Geometry check sheet. Reference: the model listing, model coordinates, mm. Face numbers are marked on the shaded views. A direction names the side the tool comes from. Give positions to 0.01 mm unless a question says otherwise; leave off trailing zeros. Order: outer loops, then holes, each group sorted by start corner. A loop starts at its lowest first (then second) coordinate and runs counter-clockwise, first axis right, second up. Notation, with made-up numbers: M 34.5,36 L 66.5,36 A32 cw 66.5,73 Z; hole C 9.25,59.5 d1. An arc over 180 degrees is marked long. One line per question, with ' | ' between items. Start each with the question number.
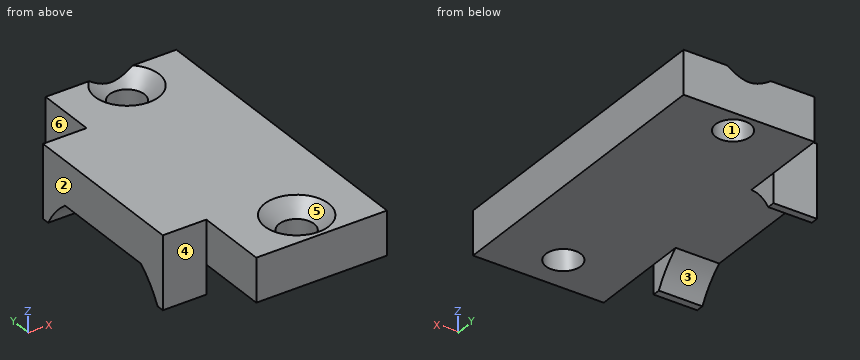
from build123d import *

# Parameters (mm, degrees)
SKETCH1_W                                       = 9
SKETCH1_H                                       = 22
BOSS_EXTRUDE1_DEPTH                             = 3
CSK_FOR_M2_FLAT_HEAD_MACHINE_SCREW1_D           = 2.4
CSK_FOR_M2_FLAT_HEAD_MACHINE_SCREW1_DEPTH       = 10
CSK_FOR_M2_FLAT_HEAD_MACHINE_SCREW1_CSINK_D     = 4.4
CSK_FOR_M2_FLAT_HEAD_MACHINE_SCREW1_CSINK_ANGLE = 90
CSK_FOR_M2_FLAT_HEAD_MACHINE_SCREW1_TIP         = 0.721032743
BOSS_EXTRUDE2_DEPTH                             = 3
SKETCH5_W                                       = 9
SKETCH5_H                                       = 3
CUT_EXTRUDE1_DEPTH                              = 0.9


with BuildPart() as part:
    # Sketch1 → Boss-Extrude1 (new body)
    with BuildSketch(Plane.XY):
        Rectangle(SKETCH1_W, SKETCH1_H)
    extrude(amount=BOSS_EXTRUDE1_DEPTH)

    # CSK for M2 Flat Head Machine Screw1
    with Locations(Plane.XY.offset(3)):
        with Locations((0, 8.5), (0, -8.5)):
            CounterSinkHole(CSK_FOR_M2_FLAT_HEAD_MACHINE_SCREW1_D / 2, CSK_FOR_M2_FLAT_HEAD_MACHINE_SCREW1_CSINK_D / 2, depth=CSK_FOR_M2_FLAT_HEAD_MACHINE_SCREW1_DEPTH, counter_sink_angle=CSK_FOR_M2_FLAT_HEAD_MACHINE_SCREW1_CSINK_ANGLE)
            with Locations((0, 0, -(CSK_FOR_M2_FLAT_HEAD_MACHINE_SCREW1_DEPTH + CSK_FOR_M2_FLAT_HEAD_MACHINE_SCREW1_TIP / 2))):  # 118° drill point
                Cone(0, CSK_FOR_M2_FLAT_HEAD_MACHINE_SCREW1_D / 2, CSK_FOR_M2_FLAT_HEAD_MACHINE_SCREW1_TIP, mode=Mode.SUBTRACT)

    # Sketch4 → Boss-Extrude2 (add)
    with BuildSketch(Plane.ZY.offset(4.5)):
        with BuildLine():
            Line((3, 6), (-2, 6))
            Line((-2, 6), (-2, 5.479963504))
            ThreePointArc((-2, 5.479963504), (-0.910429195, 4.745874502), (0, 3.798683983))
            Line((0, 3.798683983), (0, -3.798683983))
            ThreePointArc((0, -3.798683983), (-0.910429195, -4.745874502), (-2, -5.479963504))
            Line((-2, -5.479963504), (-2, -6))
            Line((-2, -6), (3, -6))
            Line((3, -6), (3, 6))
        make_face()
    extrude(amount=BOSS_EXTRUDE2_DEPTH)

    # Sketch5 → Cut-Extrude1 (cut)
    with BuildSketch(Plane(origin=(0, 11, 0), x_dir=(1, 0, 0), z_dir=(0, 1, 0))):
        with Locations((0, -1.5)):
            Rectangle(SKETCH5_W, SKETCH5_H)
    extrude(amount=-CUT_EXTRUDE1_DEPTH, mode=Mode.SUBTRACT)


solid = part.part
Item 1: Cross-section at B-B, the plane x = 0. Record the cut outline in (y, z).
Item 2: Cross-section at A-A, the plane y = 8.5. Record the cut outline in (x, z), plus the area to 3 significant figures.
Item 3: Mould release check, pull along X, two halves, no side actions. Record for the marked faces 1, 2 and 3: released by +X, released by -X, zero draft, split by the parting line, or undercut.
Item 4: Material ranges on line 1 along Y through (x, z) = (0, 1.2); line 2 along Y through (x, z) = (-1, 1.9); line 3 along X through (y, z) = (-8.5, 0.5), recorded low to high.
Item 5: Set-up check for the marked faces 4, 5 and 6: record each of +Z, -Z, +X, -X, +Y, -Y from which the full face is reachable in a straight line by a thin tool's end or side.
Item 6: Cross-section at C-C, the plane z = -1.3. Record the cut outline in (x, y).
Item 7: Depth check by flat-ended pin: pin 1 (1 mm diameter, centred on y = 5, z = -1, fed in from +X); pin 2 (1.5 mm diameter, centred on x = -1, z = -1.5, fed in from -Y); pin 3 (0.9 mm diameter, centred on x = -6, z = 0.5, fed in from -Y); pin 4 (5 mm diameter, centred on x = -1.5, y = 5, fed in from -Z). Enter the tip coordinate at first touch or a pass-through.
Item 8: Cross-section at D-D, the plane x = -5. Record the cut outline in (y, z).
Outcome:
1) outline: M -11,0 L -9.7,0 L -9.7,2 L -10.7,3 L -11,3 Z; M -7.3,0 L 7.3,0 L 7.3,2 L 6.3,3 L -6.3,3 L -7.3,2 Z; M 9.7,0 L 10.1,0 L 10.1,2.4 L 9.7,2 Z
2) outline: M -4.5,0 L -1.2,0 L -1.2,2 L -2.2,3 L -4.5,3 Z; M 1.2,0 L 4.5,0 L 4.5,3 L 2.2,3 L 1.2,2 Z | area: 18.8 mm²
3) face 1: undercut | face 2: released by -X | face 3: zero draft
4) line 1: y = -11 to -9.7, -7.3 to 7.3, 9.7 to 10.1 | line 2: y = -11 to -9.16, -7.84 to 7.84, 9.16 to 10.1 | line 3: x = -4.5 to -1.2, 1.2 to 4.5
5) face 4: +Z, -Z, -X, -Y | face 5: +Z | face 6: +Z, -Z, -X, +Y
6) outline: M -7.5,-6 L -4.5,-6 L -4.5,-5.05 L -7.5,-5.05 Z; M -7.5,5.05 L -4.5,5.05 L -4.5,6 L -7.5,6 Z
7) pin 1: stops at x = -4.5 | pin 2: passes through | pin 3: stops at y = -6 | pin 4: stops at z = 0
8) outline: M -6,-2 L -5.48,-2 A6.2 cw -3.8,0 L 3.8,0 A6.2 cw 5.48,-2 L 6,-2 L 6,3 L -6,3 Z
